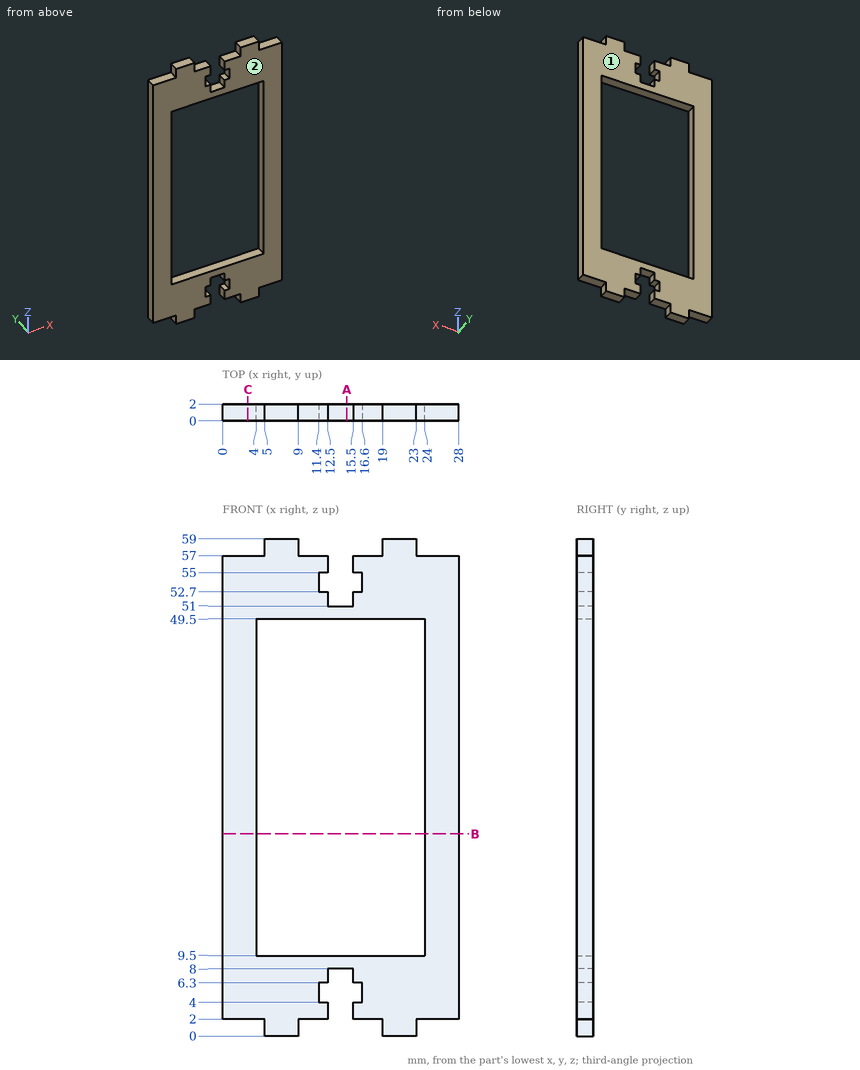
Drawing for the job (mm, zero at the part's lowest x, y, z). Give positions to 0.01 mm unless a question says otherwise; leave off trailing zeros. Write each loop counter-clockwise with the first axis right and the second up, starting at its lowest first coordinate (ties: lowest second). Pieces come first, ordered by that corner, then holes. Notation, with made-up numbers: M -36.75,-36.75 L 15.25,-36.75 A13 cw 15.25,-12.75 Z; hole C -25.5,42 d4. An arc over 180 degrees is marked long. Use CSV: the item, a comma, the result in double quotes.
Item 1: Slice it at C-C on x = 3. Write the cut outline in (y, z).
Taken from the geometry:
outline,"M 0,2 L 2,2 L 2,57 L 0,57 Z"
Item 2: Drill centre lines: probe 1 along Z at (x, y) = (19.5, 1.85); probe 2 along Z at (x, y) = (11, 1.8); probe 3 along X at (y, z) = (0.6, 38). Where is each one in solid material? Low to high.
Taken from the geometry:
probe 1,"z = 0 to 9.5, 49.5 to 59"
probe 2,"z = 2 to 9.5, 49.5 to 57"
probe 3,"x = 0 to 4, 24 to 28"
Item 3: Slice it at A-A on x = 14.75. Write the cut outline in (y, z), plus the area to 3 significant figures.
Taken from the geometry:
outline,"M 0,8 L 2,8 L 2,9.5 L 0,9.5 Z; M 0,49.5 L 2,49.5 L 2,51 L 0,51 Z"
area,"6.00 mm²"
Item 4: Pull direction Y, two halves, no side cores. Call the marked faces 1 and 2: +Y half, -Y half, draft (parallel to the pull), parting line (faces both ways), or undercut.
Taken from the geometry:
face 1,"+Y half"
face 2,"-Y half"
Item 5: Slice it at B-B on z = 24. Write the cut outline in (x, y), plus the area to 3 significant figures.
Taken from the geometry:
outline,"M 0,0 L 4,0 L 4,2 L 0,2 Z; M 24,0 L 28,0 L 28,2 L 24,2 Z"
area,"16.0 mm²"
Item 6: Pin check, flat tips, straight feed: P1, Ø0.6, axis at x = 13.5, y = 1.5, coming from the +Z side; P2, Ø0.6, axis at y = 1, z = 58, coming from the +X side; P3, Ø0.5, axis at y = 1, z = 51.5, coming from the -X side; P4, Ø0.5, axis at x = 11.5, y = 0.5, coming from the -Z side. Stop position of each tip, or through.
Taken from the geometry:
P1,"stops at z = 51"
P2,"stops at x = 23"
P3,"stops at x = 0"
P4,"stops at z = 2"
